from build123d import *

# Parameters (mm, degrees)
CROQUIS1_R                     = 19
SALIENTE_EXTRUIR1_DEPTH        = 33
CROQUIS2_R                     = 10
SALIENTE_EXTRUIR2_DEPTH        = 5
CROQUIS4_R                     = 3
SALIENTE_EXTRUIR3_DEPTH        = 12.5
SALIENTE_EXTRUIR4_REACH        = 67.204
SALIENTE_EXTRUIR4_START_RADIUS = 19
SALIENTE_EXTRUIR4_END_RADIUS   = 19


with BuildPart() as part:
    # Croquis1 → Saliente-Extruir1 (new body)
    with BuildSketch(Plane(origin=(0, 0, 0), x_dir=(1, 0, 0), z_dir=(0, 1, 0))):
        with Locations(Location((0, 0, 0), (0, 0, 270))):
            Circle(CROQUIS1_R)
    extrude(amount=SALIENTE_EXTRUIR1_DEPTH)

    # Croquis2 → Saliente-Extruir2 (add)
    with BuildSketch(Plane(origin=(0, 33, 0), x_dir=(1, 0, 0), z_dir=(0, 1, 0))):
        with Locations(Location((0, 0, 0), (0, 0, 270))):
            Circle(CROQUIS2_R)
    extrude(amount=SALIENTE_EXTRUIR2_DEPTH)

    # Croquis4 → Saliente-Extruir3 (add)
    with BuildSketch(Plane(origin=(0, 38, 0), x_dir=(1, 0, 0), z_dir=(0, 1, 0))):
        with Locations(Location((0, 0, 0), (0, 0, 270))):
            Circle(CROQUIS4_R)
    extrude(amount=SALIENTE_EXTRUIR3_DEPTH)

    # Saliente-Extruir4: from a cylinder face, 67.204 long prism both ways, kept between that surface and its translate by the depth
    saliente_extruir4_start = Plane(origin=(0, 12, 0), z_dir=(0, -1, 0)) * Cylinder(SALIENTE_EXTRUIR4_START_RADIUS, 173.408, mode=Mode.PRIVATE)
    saliente_extruir4_end = Plane(origin=(0, 12, 8), z_dir=(0, -1, 0)) * Cylinder(SALIENTE_EXTRUIR4_END_RADIUS, 173.408, mode=Mode.PRIVATE)
    # Croquis6 → Saliente-Extruir4 (add, from a surface)
    with BuildSketch(Plane.XY, mode=Mode.PRIVATE) as saliente_extruir4_sk1:
        Polygon((-5.196152423, 15), (-5.196152423, 9), (0, 6), (5.196152423, 9), (5.196152423, 15), (0, 18), align=None)
    saliente_extruir4_tool1 = extrude(saliente_extruir4_sk1.sketch, amount=SALIENTE_EXTRUIR4_REACH, both=True, mode=Mode.PRIVATE)
    add(((saliente_extruir4_tool1 - saliente_extruir4_start) & saliente_extruir4_end).solids().sort_by_distance((0, 12, 22.637833))[0])


solid = part.part
Geometry check sheet. Reference: the model listing, model coordinates, mm. A direction names the side the tool comes from. Coordinates: 2 decimals unless noted, no trailing zeros. Loops run counter-clockwise (first coordinate to the right, second up) from the corner with the lowest first, then second, coordinate; pieces in that order, holes last. Notation, with made-up numbers: (-33, 30) - (-11, 30) arc R30 cw to (-11, 62) - close; hole circle Ø4 at (-39.75, 69.5). An arc over 180 degrees is marked (long way). Use one line per item in the form item = value. Start each with the question number.
Item 1: Section check A-A, the plane z = 0. Enter the section's corners in (x, y), and give its area (3 significant figures).
Item 2: Section check B-B, the plane x = 6.5. Enter the section's corners in (y, z).
Item 3: Section check D-D, the plane z = -9. Enter the section's corners in (x, y).
Item 4: Section check C-C, the plane y = 24.5. Enter the section's corners in (x, z).
Item 5: Tool access check on faces 1 (the face through (-2.6, 16.5, 22.7)), 2 (the face through (5.196, 12, 22)), 3 (the face through (2.4, 38, 2.1)), 4 (the face through (-2.6, 7.5, 22.7)), 5 (the face through (-5.196, 12, 22)). Record the directions out of +Z, -Z, +X, -X, +Y, -Y that give a thin tool (end or side, any length) a straight path to the whole face; none if there is none.
Item 6: Thickness scan on probe 1 along Y at (x, z) = (-5, 12); probe 2 along Z at (x, y) = (16, 20); probe 3 along X at (y, z) = (9, 2). Record the ranges inside material, lowest first.
Item 7: Gauge pin test, flat ends, axial feed: pin 1 (5 mm diameter, centred on y = 24, z = 11.5, fed in from +X); pin 2 (3 mm diameter, centred on y = 12, z = 22, fed in from -X); pin 3 (1 mm diameter, centred on x = 14, z = 0, fed in from +Y). Record the tip position at first contact, or that the pin passes through.
Computed:
q1.outline = (-19, 0) - (19, 0) - (19, 33) - (10, 33) - (10, 38) - (3, 38) - (3, 50.5) - (-3, 50.5) - (-3, 38) - (-10, 38) - (-10, 33) - (-19, 33) - close
q1.area = 1,430 mm2
q2.outline = (0, -17.85) - (33, -17.85) - (33, -7.6) - (38, -7.6) - (38, 7.6) - (33, 7.6) - (33, 17.85) - (0, 17.85) - close
q3.outline = (-16.73, 0) - (16.73, 0) - (16.73, 33) - (4.36, 33) - (4.36, 38) - (-4.36, 38) - (-4.36, 33) - (-16.73, 33) - close
q4.outline = circle Ø38 at (0, 0)
q5.face_1 = +Z, -X, +Y
q5.face_2 = +Z, +X, +Y, -Y
q5.face_3 = +Y
q5.face_4 = +Z, -X, -Y
q5.face_5 = +Z, -X, +Y, -Y
q6.probe_1 = 0 to 33
q6.probe_2 = -10.25 to 10.25
q6.probe_3 = -18.89 to 18.89
q7.pin_1 = 16.73
q7.pin_2 = -5.2
q7.pin_3 = 33
